Here's how the part is built. I have some questions about the finished solid (model axes, mm). A direction names the side the tool comes from. Give positions to 0.01 mm unless a question says otherwise; leave off trailing zeros. Write each loop counter-clockwise with the first axis right and the second up, starting at its lowest first coordinate (ties: lowest second). Pieces come first, ordered by that corner, then holes. Notation, with made-up numbers: M 80.5,-21.75 L 95.5,-21.75 A7 cw 95.5,-11.75 Z; hole C 55,60.5 d6. An arc over 180 degrees is marked long. Answer as CSV lines item,"result". Start each with the question number.
Q1. Suppose I cut it at A-A (z = 3.75). Count the separate pieces of the cut face and the enclosed holes in it, then the cut area to 3 significant figures.
Q2. If I drill on line 1 along X through (y, z) = (4, 4.5); line 2 along Y through (x, z) = (-5, 0.5); line 3 along Y through (x, z) = (32, 2.5), over which ranges is the centre line in solid material (lowest first)?
Q3. On a 3-axis mill with a long thin cutter (end or side, diameter ignored), from which of +Z, -Z, +X, -X, +Y, -Y can I reach the whole of each face in a straight line? I mean faces 5 (the flat face through (-22, -10, 1.27)), 6 (the flat face through (-24, -8, 6.35)), 7 (the flat face through (-24.85, -2.208, 3.846)), 8 (the flat face through (-7.45, -10.11, 3.85)), 9 (the cylindrical face through (17.05, 1.536, 3.131)). Say none if no direction works.
Q4. Suppose I cut it at C-C (x = 25.5). Write out the boundary of the cut face in (y, z), then the cut area to 3 significant figures.
Q5. Suppose I cut it at B-B (y = -0.5). Write out the boundary of the cut face in (x, z).
Q6. Thinking about a two-plate mould opening in X: for faces 1 (the flat face through (-16, -13, 1.27)), 2 (the flat face through (-5.49, -7.17, 3.85)), 3 (the flat face through (12, 5, 6.35)), 4 (the cylindrical face through (-24.448, -9.979, 1.014)), which applies, +X half, -X half, draft (parallel to the pull), parting line (faces both ways), or undercut?
Q7. Suppose I cut it at D-D (x = 1). Write out the boundary of the cut face in (y, z), then the cut area to 3 significant figures.
Q8. For pin 1 (2 mm diameter, centred on x = -18.5, z = 5.5, fed in from -Y); pin 2 (3 mm diameter, centred on y = 5.5, z = 1, fed in from -X); pin 3 (2 mm diameter, centred on x = 4, z = 3, fed in from +Y); pin 4 (12 mm diameter, centred on x = 21.5, y = -7, fed in from -Z), each with a flat end and sliding along its axis, tell me the tip position at first contact or that it passes through.
```python
from build123d import *

# Parameters (mm, degrees)
F0_R     = 8.371120517
F1_DEPTH = 6.35
F4_DEPTH = 5.08
F6_DEPTH = 5.08


with BuildPart() as f1:
    # F0 (on Top) → F1 (new body)
    with BuildSketch(Plane.XY):
        with BuildLine():
            Line((38.1892591841, 8.8001990686), (-12.6107408159, 8.8001990686))
            ThreePointArc((-12.6107408159, 8.8001990686), (-24.206336891, -10.3022339435), (-2.7967678425, -3.8998009314))
            ThreePointArc((-2.7967678425, -3.8998009314), (17.3389637973, 1.581272222), (38.1892591841, 2.4501990686))
            Line((38.1892591841, 2.4501990686), (38.1892591841, 8.8001990686))
        make_face()
        with Locations((-14.7333428902, -2.9819420458)):
            Circle(F0_R, mode=Mode.SUBTRACT)
    extrude(amount=F1_DEPTH)

    # F3 (on face) → F4 (cut)
    with BuildSketch(Plane.XY.offset(6.35)):
        with BuildLine():
            Line((-13.560262228, -14.8961424203), (-13.9130828172, -11.3127782657))
            ThreePointArc((-13.9130828172, -11.3127782657), (-15.3721789388, -11.3286508112), (-16.8118643504, -11.0909128344))
            Line((-16.8118643504, -11.0909128344), (-17.7059041681, -14.5788454365))
            ThreePointArc((-17.7059041681, -14.5788454365), (-15.6469631426, -14.9188422648), (-13.560262228, -14.8961424203))
        make_face()
        with BuildLine():
            Line((-6.1764105875, -11.3547073221), (-8.7500289189, -8.8364798269))
            ThreePointArc((-8.7500289189, -8.8364798269), (-9.8575587193, -9.7865278105), (-11.1132367545, -10.5298218989))
            Line((-11.1132367545, -10.5298218989), (-9.5561111287, -13.7764110041))
            ThreePointArc((-9.5561111287, -13.7764110041), (-7.7603250488, -12.7134019048), (-6.1764105875, -11.3547073221))
        make_face()
        with BuildLine():
            Line((-2.7877611159, -3.8962267625), (-6.3866341249, -3.6207780944))
            ThreePointArc((-6.3866341249, -3.6207780944), (-6.6243721016, -5.060463506), (-7.1084970525, -6.4369940948))
            Line((-7.1084970525, -6.4369940948), (-3.828802369, -7.9231245789))
            ThreePointArc((-3.828802369, -7.9231245789), (-3.1369674478, -5.9565622573), (-2.7967678425, -3.8998009314))
            ThreePointArc((-2.7967678425, -3.8998009314), (-2.7922645256, -3.89801373), (-2.7877611159, -3.8962267625))
        make_face()
        with BuildLine():
            Line((-21.4930113477, -12.8627907518), (-19.4599455199, -9.8909858503))
            ThreePointArc((-19.4599455199, -9.8909858503), (-20.5878806714, -8.9652560172), (-21.5379286549, -7.8577262167))
            Line((-21.5379286549, -7.8577262167), (-24.4648027493, -9.9549598872))
            ThreePointArc((-24.4648027493, -9.9549598872), (-23.1061081665, -11.5388743485), (-21.4930113477, -12.8627907518))
        make_face()
        with BuildLine():
            Line((-26.2628364708, -6.2060801603), (-22.7951783218, -5.2363750533))
            ThreePointArc((-22.7951783218, -5.2363750533), (-23.0641791102, -3.8022021189), (-23.0800516556, -2.3431059972))
            Line((-23.0800516556, -2.3431059972), (-26.6702431093, -2.0683217935))
            ThreePointArc((-26.6702431093, -2.0683217935), (-26.6475432648, -4.155022708), (-26.2628364708, -6.2060801603))
        make_face()
        with BuildLine():
            ThreePointArc((-22.358188728, 0.4731100032), (-21.6423866947, 1.7446605838), (-20.7166568616, 2.8725957353))
            Line((-20.7166568616, 2.8725957353), (-23.2902751929, 5.3908232305))
            ThreePointArc((-23.2902751929, 5.3908232305), (-24.6141915962, 3.7777264117), (-25.6378834115, 1.9592404873))
            Line((-25.6378834115, 1.9592404873), (-22.358188728, 0.4731100032))
        make_face()
        with BuildLine():
            ThreePointArc((-18.353449026, 4.5659378073), (-16.9877758977, 5.0798933858), (-15.5536029633, 5.3488941741))
            Line((-15.5536029633, 5.3488941741), (-15.9064235525, 8.9322583287))
            ThreePointArc((-15.9064235525, 8.9322583287), (-17.9574810047, 8.5475515347), (-19.9105746518, 7.8125269125))
            Line((-19.9105746518, 7.8125269125), (-18.353449026, 4.5659378073))
        make_face()
    extrude(amount=-F4_DEPTH, mode=Mode.SUBTRACT)

    # F5 (on face) → F6 (cut)
    with BuildSketch(Plane.XY.offset(6.35)):
        with BuildLine():
            ThreePointArc((-15.4898996277, 5.2621371657), (-8.9244307049, 2.9166814686), (-6.4786379033, -3.6120735562))
            Line((-6.4786379033, -3.6120735562), (-6.4786379033, -3.865575185))
            Line((-6.4786379033, -3.865575185), (-2.7950332078, -4.1475090028))
            Line((-2.7950332078, -4.1475090028), (-2.7950332078, -3.894007374))
            ThreePointArc((-2.7950332078, -3.894007374), (-6.3406722718, 5.5572722698), (-15.8519057587, 8.9387927615))
            Line((-15.8519057587, 8.9387927615), (-16.2552728318, 8.8990769519))
            Line((-16.2552728318, 8.8990769519), (-15.8971771478, 5.2621371657))
            Line((-15.8971771478, 5.2621371657), (-15.4898996277, 5.2621371657))
        make_face()
    extrude(amount=-F6_DEPTH, mode=Mode.SUBTRACT)


solid = f1.part
```
Resolved:
1,separate pieces,"7"
1,enclosed holes,"0"
1,area,"431 mm^2"
2,line 1,"-21.87 to -19.35, -5.01 to 38.19"
2,line 2,"-9.95 to 8.8"
2,line 3,"2.68 to 8.8"
3,face 5,"+Z"
3,face 6,"+Z, +X, -X, +Y, -Y"
3,face 7,"+Z, -X"
3,face 8,"+Z, -Y"
3,face 9,"+Z, -Z, -Y"
4,outline,"M 2.48,0 L 8.8,0 L 8.8,6.35 L 2.48,6.35 Z"
4,area,"40.1 mm^2"
5,outline,"M -26.45,0 L -22.73,0 L -22.73,6.35 L -26.45,6.35 Z; M -6.74,0 L 7.47,0 L 7.47,6.35 L -3.02,6.35 L -3.02,1.27 L -6.74,1.27 Z"
6,face 1,"undercut"
6,face 2,"+X half"
6,face 3,"draft"
6,face 4,"parting line"
7,outline,"M -2.49,0 L 8.8,0 L 8.8,6.35 L -2.49,6.35 Z"
7,area,"71.7 mm^2"
8,pin 1,"y = -14.58"
8,pin 2,"x = -24.46"
8,pin 3,"y = 8.8"
8,pin 4,"through"
